Geometry: final body of the model. Coordinates: model frame, mm. Round coordinates to 2 decimals unless told otherwise and drop trailing zeros. Loops run counter-clockwise (first coordinate to the right, second up) from the corner with the lowest first, then second, coordinate; pieces in that order, holes last. Notation, with made-up numbers: (-35.5, 56.5) - (17.5, 56.5) arc R4 ccw to (17.5, 63.5) - close; hole circle Ø10 at (2.25, -16.5). An arc over 180 degrees is marked (long way). Answer as a JSON object with one key per item and string values. Group by question number.
Item 1: Line query: line 1 (Z direction, x = 8.5, y = 2); line 2 (Y direction, x = -15.5, z = 10.5); line 3 (X direction, y = 9.75, z = 6). Output: solid intervals per line, ascending.
Item 2: First-contact query: pin 1 (8 mm diameter, centred on x = -1, y = 7, fed in from -Z). Flat tip, straight axial feed; report the tip coordinate or a pass-through.
Item 3: Section B-B (y = 0.5). Return the cut outline in (x, z).
Item 4: Section A-A (z = 37). Return the cut outline in (x, y), plus the area to 3 significant figures.
```python
from build123d import *

# Parameters (mm, degrees)
F1_DEPTH = 50
F2_W     = 5
F2_H     = 12.5
F3_DEPTH = 10


with BuildPart() as f1:
    # F0 (on Top) → F1 (new body)
    with BuildSketch(Plane.XY):
        with BuildLine():
            Line((-15.25, -10.75), (15.25, -10.75))
            ThreePointArc((15.25, -10.75), (17.017767, -10.017767), (17.75, -8.25))
            Line((17.75, -8.25), (17.75, 8.25))
            ThreePointArc((17.75, 8.25), (17.017767, 10.017767), (15.25, 10.75))
            Line((15.25, 10.75), (-15.25, 10.75))
            ThreePointArc((-15.25, 10.75), (-17.017767, 10.017767), (-17.75, 8.25))
            Line((-17.75, 8.25), (-17.75, -8.25))
            ThreePointArc((-17.75, -8.25), (-17.017767, -10.017767), (-15.25, -10.75))
        make_face()
    extrude(amount=F1_DEPTH)

    # F2 (on face) → F3 (cut)
    with BuildSketch(Plane.YZ.offset(17.75)):
        with Locations((0, 35.25)):
            Rectangle(F2_W, F2_H)
    extrude(amount=-F3_DEPTH, mode=Mode.SUBTRACT)


solid = f1.part
```
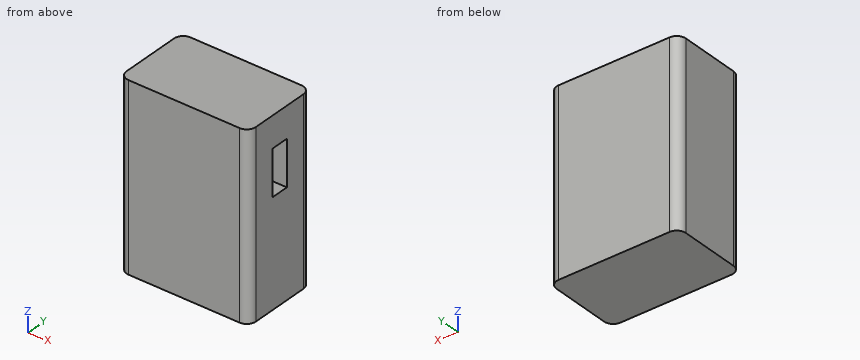
Values:
{
 "1": {"line 1": "z = 0 to 29, 41.5 to 50", "line 2": "y = -10.74 to 10.74", "line 3": "x = -17.25 to 17.25"},
 "2": {"pin 1": "stops at z = 0"},
 "3": {"outline": "(-17.75, 0) - (17.75, 0) - (17.75, 29) - (7.75, 29) - (7.75, 41.5) - (17.75, 41.5) - (17.75, 50) - (-17.75, 50) - close"},
 "4": {"outline": "(-17.75, -8.25) arc R2.5 ccw to (-15.25, -10.75) - (15.25, -10.75) arc R2.5 ccw to (17.75, -8.25) - (17.75, -2.5) - (7.75, -2.5) - (7.75, 2.5) - (17.75, 2.5) - (17.75, 8.25) arc R2.5 ccw to (15.25, 10.75) - (-15.25, 10.75) arc R2.5 ccw to (-17.75, 8.25) - close", "area": "708 mm^2"}
}
